Study the drawing (mm; zero at the part's minimum x, y, z) and answer. Round coordinates to 2 decimals unless told otherwise and drop trailing zeros. Write each loop counter-clockwise with the first axis right and the second up, starting at its lowest first coordinate (ties: lowest second). Pieces come first, ordered by that corner, then holes. Notation, with made-up numbers: (26.25, 33) - (61.25, 33) arc R10 cw to (61.25, 39) - close; hole circle Ø9 at (48, -28.75). An arc over 180 degrees is marked (long way). Use one line per item in the form item = value. Start each with the question number.
1) The part is cut by section A-A, the plane y = 6. Give the vertices of the cut face in (x, z), plus the area to 3 significant figures.
2) Consider line 1 along Y through (x, z) = (6, 1.25); line 2 along Y through (x, z) = (8.75, 0.95); line 3 along X through (y, z) = (4.25, 0.85). Determine where each line is inside the solid, lowest interval first. Write a range as from..to.
3) For a pull along X with two mould halves and no side action, classify the marked faces 1, 2 and 3 as released by +X, released by -X, zero draft, split by the parting line, or undercut.
4) The part is cut by section C-C, the plane z = 1. Give the vertices of the cut face in (x, y).
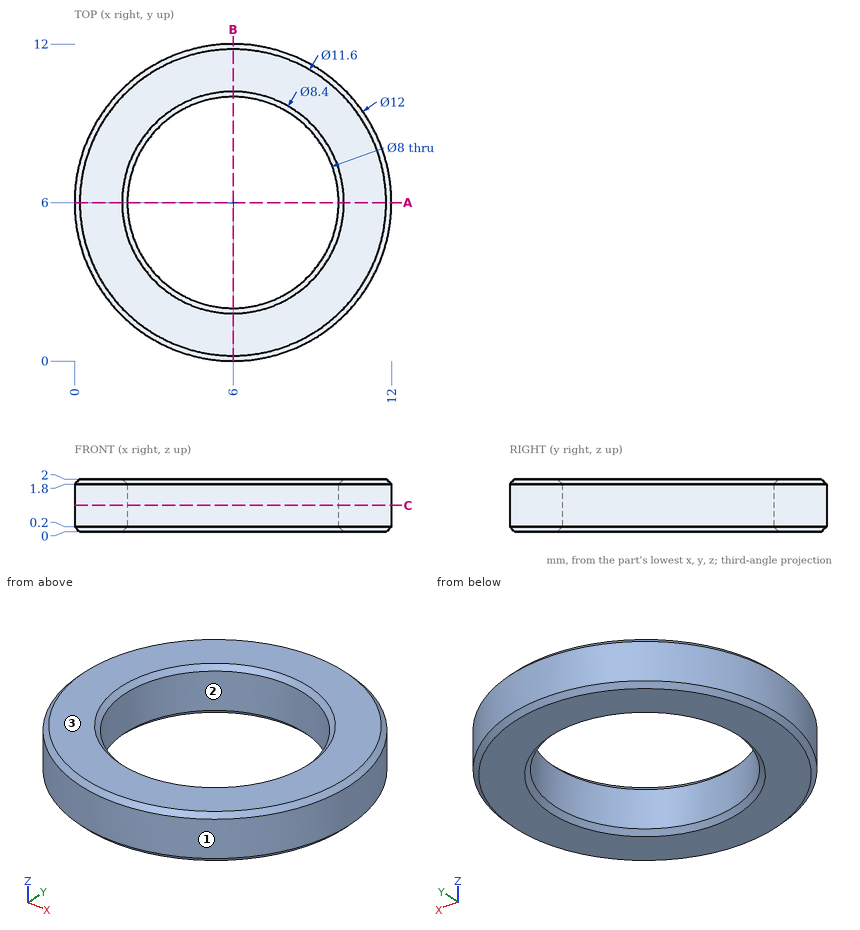
Geometry results:
q1.outline = (0, 0.2) - (0.2, 0) - (1.8, 0) - (2, 0.2) - (2, 1.8) - (1.8, 2) - (0.2, 2) - (0, 1.8) - close; (10, 0.2) - (10.2, 0) - (11.8, 0) - (12, 0.2) - (12, 1.8) - (11.8, 2) - (10.2, 2) - (10, 1.8) - close
q1.area = 7.84 mm2
q2.line_1 = 0..2, 10..12
q2.line_2 = 0.67..3.1, 8.9..11.33
q2.line_3 = 0.26..2.4, 9.6..11.74
q3.face_1 = split by the parting line
q3.face_2 = undercut
q3.face_3 = zero draft
q4.outline = circle Ø12 at (6, 6); hole circle Ø8 at (6, 6)
